Autodesk Inventor part; units mm, degrees
ref_plane "YZ Plane" through (0, 0, 0) normal (1, 0, 0) x (0, 1, 0)
ref_plane "XZ Plane" through (0, 0, 0) normal (0, 1, 0) x (-1, 0, 0)
ref_plane "XY Plane" through (0, 0, 0) normal (0, 0, 1) x (1, 0, 0)
sketch "Esboço1" plane through (0, 0, 0) normal (0, 0, 1) x (1, 0, 0)
  circle A0 centre (0, 0) radius 8
  dimension "d0" = 16
extrude "Extrusão1" add sketch "Esboço1" along normal blind 235
sketch "Esboço2" plane through (0, 0, 235) normal (0, 0, 1) x (1, 0, 0)
  circle A0 centre (0, 0) radius 6
  dimension "d3" = 12
extrude "Extrusão2" add sketch "Esboço2" along normal blind 39
sketch "Esboço3" plane through (0, 0, 274) normal (0, 0, 1) x (1, 0, 0)
  circle A0 centre (0, 0) radius 5
  dimension "d6" = 10
extrude "Extrusão3" add sketch "Esboço3" along normal blind 15
sketch "Esboço4" plane through (0, 0, 0) normal (0, 0, -1) x (-1, 0, 0)
  circle A0 centre (0, 0) radius 5
  dimension "d9" = 10
extrude "Extrusão4" add sketch "Esboço4" along normal blind 9.15
sketch "Esboço5" plane through (0, 0, -9.15) normal (0, 0, -1) x (-1, 0, 0)
  circle A0 centre (0, 0) radius 4.5
  dimension "d12" = 9
extrude "Extrusão5" add sketch "Esboço5" along normal blind 1.15
sketch "Esboço6" plane through (0, 0, -10.3) normal (0, 0, -1) x (-1, 0, 0)
  circle A0 centre (0, 0) radius 5
  dimension "d15" = 10
extrude "Extrusão6" add sketch "Esboço6" along normal blind 1.85
thread "Rosca1"
chamfer "Chanfro1" distance 0.5 angle 45 5 edges at (-5, 0, 289) (-6, 0, 274) (-8, 0, 235) (-8, 0, 0) (5, 0, -12.15)
properties part number "SFU16XX_Z"
Geometry: final body of the model. Coordinates: model frame, mm. A direction names the side the tool comes from. Coordinates: 2 decimals unless noted, no trailing zeros. Order: outer loops, then holes, each group sorted by start corner. A loop starts at its lowest first (then second) coordinate and runs counter-clockwise, first axis right, second up.
Item 1: Material intervals for line 1 along X through (y, z) = (5.25, 179); line 2 along X through (y, z) = (5.75, 225); line 3 along Y through (x, z) = (-0.5, 93.5), sorted ascending.
Answer:
line 1: x = -6.04 to 6.04
line 2: x = -5.56 to 5.56
line 3: y = -7.98 to 7.98
Item 2: Access query for faces 4 (the face through (-1.73, 7.81, 115.86)), 5 (the face through (2, 6, 235)), 6 (the face through (1.08, 4.88, -10.97)). Directions: +Z, -Z, +X, -X, +Y, -Y. A direction counts if a zero-diameter tool reaches every point of the face in a straight line with its end or side. Return the directions, or none.
Answer:
face 4: +Z, -Z
face 5: +Z
face 6: -Z
Item 3: Section query C-C (z = 155.5). Output: boundary loops of the cut face in (x, y), then the cut area to 3 significant figures.
Answer:
outline: circle Ø16 at (0, 0)
area: 201 mm2
Item 4: Contact query for flat-ended pins moving along their axis: P1, Ø1, axis at y = 5, z = 246, coming from the +X side; P2, Ø6, axis at y = 0.5, z = 249.5, coming from the +X side; P3, Ø6, axis at y = -5, z = 148.5, coming from the +X side. Output: stop coordinate, or through.
Answer:
P1: stops at x = 3.97
P2: stops at x = 6
P3: stops at x = 7.75
Item 5: Draft query along Z for faces 1 (the face through (0, 0, -12.15)), 2 (the face through (-1.08, 4.88, 281.15)), 3 (the face through (0.59, -4.46, -9.72)). Return one class per face: released by +Z, released by -Z, zero draft, split by the parting line, or undercut.
Answer:
face 1: released by -Z
face 2: zero draft
face 3: undercut
